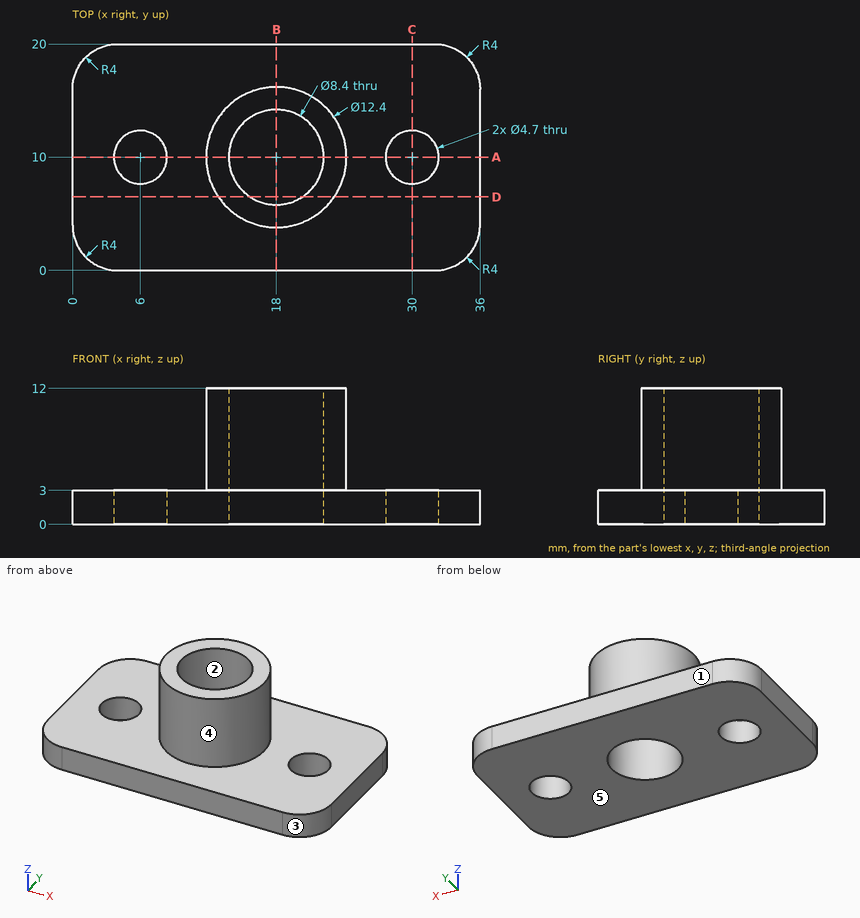
Check sheet for the drawn part. Datum: minimum x, y, z corner. Units: mm. A direction names the side the tool comes from. Round coordinates to 2 decimals unless told otherwise and drop trailing zeros. Order: outer loops, then holes, each group sorted by start corner. A loop starts at its lowest first (then second) coordinate and runs counter-clockwise, first axis right, second up. Notation, with made-up numbers: (5, -29) -> (29, -29) arc R36 ccw to (29, 5) -> close; hole circle Ø2 at (-27, 75). An arc over 180 degrees is marked (long way). Put each result on its own line as item: value. Start each with the question number.
(1) Section check B-B (x = 18). Enter the section's corners in (y, z), then the cut area to 3 significant figures.
(2) Material ranges on line 1 along Y through (x, z) = (18, 4.75); line 2 along Y through (x, z) = (6, 1.9); line 3 along Z through (x, y) = (34, 18.5), recorded low to high.
(3) Section check C-C (x = 30). Enter the section's corners in (y, z).
(4) Section check D-D (y = 6.5). Enter the section's corners in (x, z).
(5) Draft check along Y on the marked faces 1, 2 and 3. Enter one of: +Y half, -Y half, draft (parallel to the pull), parting line (faces both ways), or undercut.
(6) Tool access check on the marked faces 4 and 5. Record the directions out of +Z, -Z, +X, -X, +Y, -Y that give a thin tool (end or side, any length) a straight path to the whole face; none if there is none.
(7) Depth check by flat-ended pin: pin 1 Ø6 at (y, z) = (11.5, 9.5) entering from +X; pin 2 Ø3 at (y, z) = (14.5, 3) entering from -X; pin 3 Ø5.5 at (x, y) = (30, 10) entering from +Z; pin 4 Ø6.5 at (x, y) = (18, 10) entering from +Z. Enter the tip coordinate at first touch or a pass-through.
(8) Section check A-A (y = 10). Enter the section's corners in (x, z).
Completed:
1. outline: (0, 0) -> (5.8, 0) -> (5.8, 12) -> (3.8, 12) -> (3.8, 3) -> (0, 3) -> close; (14.2, 0) -> (20, 0) -> (20, 3) -> (16.2, 3) -> (16.2, 12) -> (14.2, 12) -> close
1. area: 70.8 mm2
2. line 1: y = 3.8 to 5.8, 14.2 to 16.2
2. line 2: y = 0 to 7.65, 12.35 to 20
2. line 3: z = 0 to 3
3. outline: (0, 0) -> (7.65, 0) -> (7.65, 3) -> (0, 3) -> close; (12.35, 0) -> (20, 0) -> (20, 3) -> (12.35, 3) -> close
4. outline: (0, 0) -> (15.68, 0) -> (15.68, 12) -> (12.88, 12) -> (12.88, 3) -> (0, 3) -> close; (20.32, 0) -> (36, 0) -> (36, 3) -> (23.12, 3) -> (23.12, 12) -> (20.32, 12) -> close
5. face 1: +Y half
5. face 2: undercut
5. face 3: -Y half
6. face 4: +Z
6. face 5: -Z, +X, -X, +Y, -Y
7. pin 1: stops at x = 24.2
7. pin 2: stops at x = 0
7. pin 3: stops at z = 3
7. pin 4: passes through
8. outline: (0, 0) -> (3.65, 0) -> (3.65, 3) -> (0, 3) -> close; (8.35, 0) -> (13.8, 0) -> (13.8, 12) -> (11.8, 12) -> (11.8, 3) -> (8.35, 3) -> close; (22.2, 0) -> (27.65, 0) -> (27.65, 3) -> (24.2, 3) -> (24.2, 12) -> (22.2, 12) -> close; (32.35, 0) -> (36, 0) -> (36, 3) -> (32.35, 3) -> close
